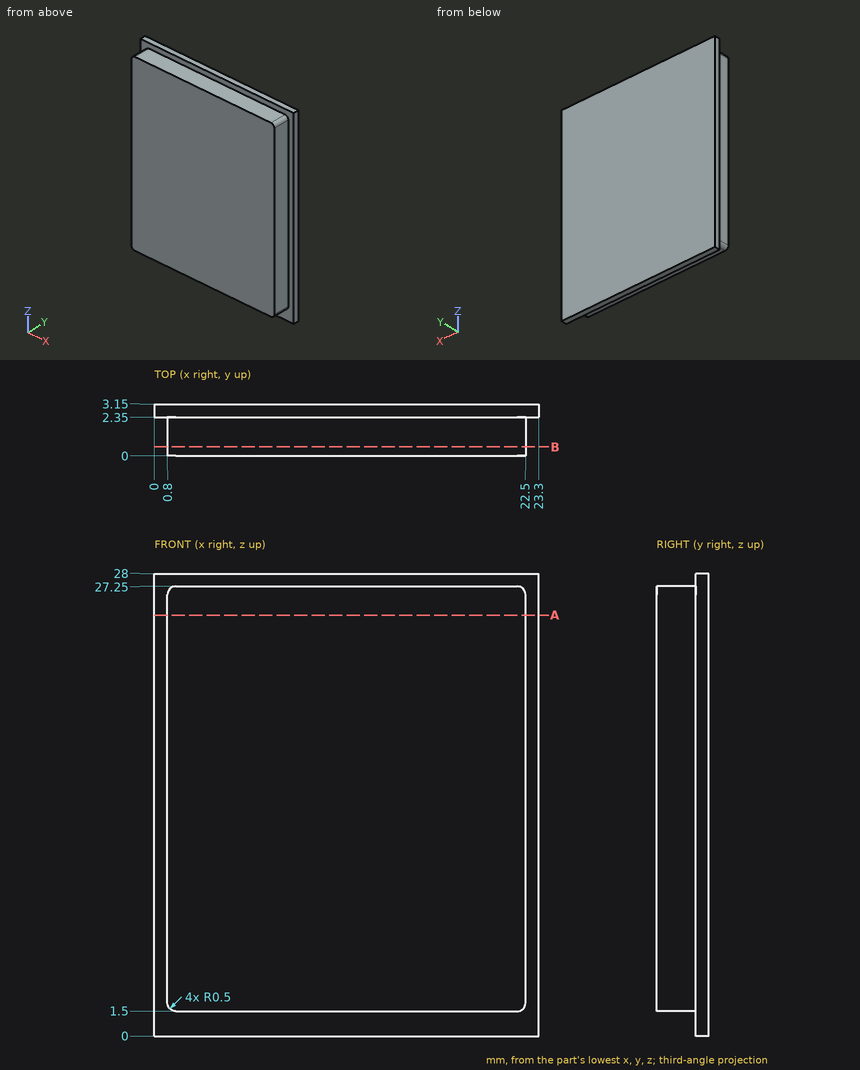
Drawing for the job (mm, zero at the part's lowest x, y, z). Give positions to 0.01 mm unless a question says otherwise; leave off trailing zeros. Order: outer loops, then holes, each group sorted by start corner. A loop starts at its lowest first (then second) coordinate and runs counter-clockwise, first axis right, second up. Notation, with made-up numbers: (72.25, -16.5) - (114.25, -16.5) arc R13 ccw to (114.25, -5.5) - close; hole circle Ø11 at (58.25, 60). An arc over 180 degrees is marked (long way). Write item = value, one per line. Start each with the question number.
1. Cut at B-B, the plane y = 0.55. List the corners of the cut face in (x, z), and give its area (3 significant figures).
2. Probe line 1 along X through (y, z) = (2, 19.75); line 2 along Z through (x, y) = (19.75, 1.75). List the from-to ranges inside material, lowest first.
3. Cut at A-A, the plane z = 25.5. List the corners of the cut face in (x, y).
4. Drop flat-ended pins along their axis: P1, Ø1.2, axis at x = 10.5, y = 1.5, coming from the -Z side; P2, Ø0.7, axis at y = 1, z = 9.5, coming from the +X side. Give the stop position or say it passes through.
Taken from the geometry:
q1.outline = (0.8, 2) arc R0.5 ccw to (1.3, 1.5) - (22, 1.5) arc R0.5 ccw to (22.5, 2) - (22.5, 26.75) arc R0.5 ccw to (22, 27.25) - (1.3, 27.25) arc R0.5 ccw to (0.8, 26.75) - close
q1.area = 559 mm²
q2.line_1 = 0.8 to 22.5
q2.line_2 = 1.5 to 27.25
q3.outline = (0, 2.35) - (0.8, 2.35) - (0.8, 0) - (22.5, 0) - (22.5, 2.35) - (23.3, 2.35) - (23.3, 3.15) - (0, 3.15) - close
q4.P1 = 1.5
q4.P2 = 22.5
